Model file for the job. Use its own axes, mm. A direction names the side the tool comes from. Round coordinates to 2 decimals unless told otherwise and drop trailing zeros. Order: outer loops, then holes, each group sorted by start corner. A loop starts at its lowest first (then second) coordinate and runs counter-clockwise, first axis right, second up. Notation, with made-up numbers: M 45.25,42 L 84.25,42 A13 ccw 84.25,48 Z; hole C -14.75,-21.5 d7. An arc over 180 degrees is marked long. Return JSON: item names as keys, results as strings. Group by question number.
Item 1: Pull direction Y, two halves, no side cores. Call faces 3 (the face through (-37.37, 11.9, -80.26)), 4 (the face through (-38.53, -9.404, -75.387)), 5 (the face through (24.2, -5.2, -113)), 6 (the face through (-18.24, -15.01, -32.76)): pulls with the +Y half, pulls with the -Y half, needs draft (parallel to the pull), parting line crosses it, or undercut.
Item 2: Slice it at A-A on z = -43. Write the cut outline in (x, y), then the cut area to 3 significant figures.
Item 3: Pin check, flat tips, straight feed: pin 1 Ø8 at (x, y) = (-0.59, -5.1) entering from +Z; pin 2 Ø2 at (x, z) = (-8.5, -61) entering from +Y; pin 3 Ø5 at (x, z) = (15, -78) entering from +Y; pin 4 Ø1 at (y, z) = (20, -76.5) entering from -X. Stop position of each tip, or through.
Item 4: Probe line 1 along X through (y, z) = (0, -101.5); line 2 along Y through (x, z) = (19.5, -99); line 3 along X through (y, z) = (-7, -62.5). List the from-to ranges inside material, lowest first.
Item 5: Which spindle directions (+Z, -Z, +X, -X, +Y, -Y) get a long thin tool onto all of the face, cutting with end or side? Do faces 1 (the face through (17.52, 20.08, -102.86)), 2 (the face through (-11.31, 12.34, -15.52)). Say none if no direction does.
from build123d import *

# Parameters (mm, degrees)
F_10_0MM_DOWEL_HOLE1_D           = 10
F_10_0MM_DOWEL_HOLE1_CSINK_D     = 10.05
F_10_0MM_DOWEL_HOLE1_CSINK_ANGLE = 90


with BuildPart() as part:
    # ff → Revolve1 (revolve)
    with BuildSketch(Plane(origin=(0, 0, 0), x_dir=(1, 0, 0), z_dir=(0, 1, 0))):
        Polygon((-27.469034289, 50), (-28.669034289, 50), (-29.932925511, 54.335656855), (-31.468331613, 57.777529323), (-33.489527061, 61.506224497), (-35.752379109, 65.81164745), (-37.618887017, 70.122472229), (-39.86237248, 75.117178167), (-41.669034289, 79.422637332), (-42.669034289, 85.208855182), (-42.669034289, 90.333303824), (-42.669034289, 93), (-42.669034289, 113), (-41.669034289, 113), (-41.669034289, 93), (-39.371495413, 77.8398126), (-34.076931722, 65.81164745), (-29.932925511, 59.326371933), (-27.094890318, 53.934105067), (-26.469034289, 50), (-26.469034289, 16), (-8.669034289, 16), (-8.669034289, 15), (-27.469034289, 15), align=None)
    revolve(axis=Axis((-8.669034289, 0, -16), (0, 0, 1)))

    # Ø10.0mm Dowel Hole1 (through all)
    with Locations(Plane.XY.offset(-15)):
        with Locations((-8.62181152, 8.122316285), (-16.271900114, -5.100059063), (-0.593940773, -5.100059063)):
            CounterSinkHole(F_10_0MM_DOWEL_HOLE1_D / 2, F_10_0MM_DOWEL_HOLE1_CSINK_D / 2, counter_sink_angle=F_10_0MM_DOWEL_HOLE1_CSINK_ANGLE)


solid = part.part
Output values:
{
 "1": {"face 3": "undercut", "face 4": "parting line crosses it", "face 5": "needs draft", "face 6": "undercut"},
 "2": {"outline": "C -8.67,0 d37.6; hole C -8.67,0 d35.6", "area": "115 mm²"},
 "3": {"pin 1": "through", "pin 2": "y = 25.08", "pin 3": "y = 24.94", "pin 4": "x = -33.84"},
 "4": {"line 1": "-42.67 to -41.67, 24.33 to 25.33", "line 2": "-19.04 to -17.19, 17.19 to 19.04", "line 3": "-33.03 to -30.88, 13.55 to 15.69"},
 "5": {"face 1": "-Z", "face 2": "+Z, -Z"}
}
